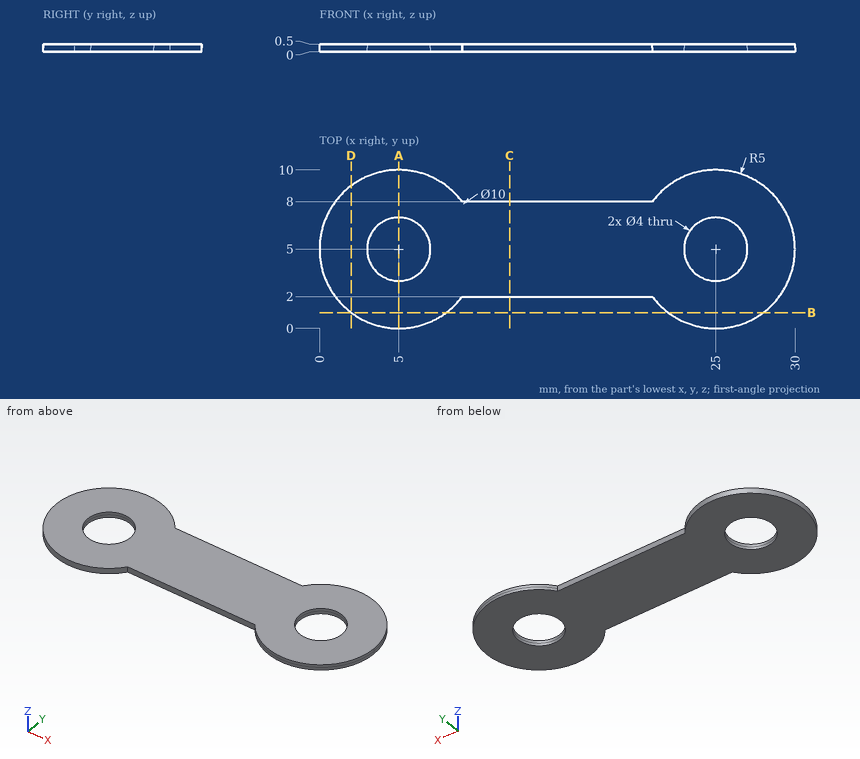
Design review of the part shown in the three views and the two pictorial views. Dimensions are in mm from the part's minimum x, y and z. Coordinates: 2 decimals unless noted, no trailing zeros. Write each loop counter-clockwise with the first axis right and the second up, starting at its lowest first coordinate (ties: lowest second). Pieces come first, ordered by that corner, then holes.
(1) Add section D-D on x = 2. Give the boundary of the cut face in (y, z), then the cut area to 3 significant figures.
(2) Add section B-B on y = 1. Give the boundary of the cut face in (x, z).
(3) Add section A-A on x = 5. Give the boundary of the cut face in (y, z).
(4) Wall thickness on probe 1 along X at (y, z) = (4.75, 0.15); probe 2 along Y at (x, z) = (25, 0.35); probe 3 along X at (y, z) = (3.25, 0.3): over which ranges is each line inside the solid? List them lowest first.
(5) Add section C-C on x = 12. Give the boundary of the cut face in (y, z).
Answer sheet:
1. outline: (1, 0) - (9, 0) - (9, 0.5) - (1, 0.5) - close
1. area: 4.00 mm2
2. outline: (2, 0) - (8, 0) - (8, 0.5) - (2, 0.5) - close; (22, 0) - (28, 0) - (28, 0.5) - (22, 0.5) - close
3. outline: (0, 0) - (3, 0) - (3, 0.5) - (0, 0.5) - close; (7, 0) - (10, 0) - (10, 0.5) - (7, 0.5) - close
4. probe 1: x = 0.01 to 3.02, 6.98 to 23.02, 26.98 to 29.99
4. probe 2: y = 0 to 3, 7 to 10
4. probe 3: x = 0.32 to 4.03, 5.97 to 24.03, 25.97 to 29.68
5. outline: (2, 0) - (8, 0) - (8, 0.5) - (2, 0.5) - close
